Autodesk Inventor part; units mm, degrees
ref_plane "Work Plane1" through (5.1, 0, 0) normal (0, 0.866, -0.5) x (-1, 0, 0)
ref_plane "YZ Plane" through (0, 0, 0) normal (1, 0, 0) x (0, 1, 0)
ref_plane "XZ Plane" through (0, 0, 0) normal (0, 1, 0) x (-1, 0, 0)
sketch "Sketch1" plane through (0, 0, 0) normal (1, 0, 0) x (0, 1, 0)
  line L0 (-4.9075, -8.5) -> (-9.815, 0)
  line L1 (-9.815, 0) -> (-4.9075, 8.5)
  line L2 (-4.9075, 8.5) -> (4.9075, 8.5)
  line L3 (4.9075, 8.5) -> (9.815, 0)
  line L4 (9.815, 0) -> (4.9075, -8.5)
  line L5 (4.9075, -8.5) -> (-4.9075, -8.5)
  point P0 (0, 0)
  point P1 (0, 0)
  dimension "d0" = 19.6299
extrude "Body" add sketch "Sketch1" along normal blind 8
sketch "Sketch2" plane through (0, 0, 0) normal (0, 0, 1) x (1, 0, 0)
  line L0 (8, 0) -> (16.5, 0)
  arc A0 (16.5, 0) -> (8, 8.5) centre (8, 0) ccw
  line L1 (8, 8.5) -> (8, 8.5)
  line L2 (8, -4.9075) -> (8, 4.9075)
  line L3 (8, 0) -> (8, 8.5)
  line L4 (5.9479, 0) -> (20.3125, 0)
  dimension "d8" = 8.5
  dimension "d9" = 8.5
revolve "Cap" add sketch "Sketch2" angle 360 about axis through (8, 0, 0) along (1, 0, 0)
sketch "Sketch3" plane through (0, 0, 0) normal (-1, 0, 0) x (0, 0, 1)
  line L0 (0, -13.7409) -> (0, 13.7409)
  line L1 (-11.9, 0) -> (11.9, 0)
  point P0 (0, 0)
hole "Thread" at (0, 0, 0) direction (1, 0, 0) diameter 8.376 depth 10.2 tip angle 120
sketch "Sketch4" plane through (0, 0, 0) normal (0, 0, 1) x (1, 0, 0)
  line L0 (0, 4.9075) -> (0, 9.815)
  line L1 (0, 9.815) -> (8, 9.815)
  line L2 (8, 4.9075) -> (8, 9.815)
  line L3 (-1.6, 0) -> (9.6, 0)
  line L4 (0.7592, 9.815) -> (0, 8.5)
  line L5 (7.2408, 9.815) -> (8, 8.5)
  dimension "d3" = 17
  dimension "d4" = 30
  dimension "d5" = 17
  dimension "d6" = 30
revolve "Chamfer1" cut sketch "Sketch4" angle 360 about axis through (-10, 0, 0) along (1, 0, 0)
chamfer "Chamfer2" distance 0.8119 angle 30 1 edges at (0, 0, -4.188) measured on face at (0, -7.0214, 0.1683)
ref_plane "Work Plane1" through (5.1, 0, 0) normal (0, 0.866, -0.5) x (-1, 0, 0)
equation "\"d0\" = 1.1547 * SW"
equation "\"d1\" = SIH"
equation "\"d8\" = KR"
equation "\"d9\" = KOH1 - SIH"
equation "\"d11\" = GEL"
equation "\"d12\" = 1.02 * GEL"
equation "\"d3\" = SW0"
equation "\"d4\" = ANG1"
equation "\"d5\" = SW01"
equation "\"d6\" = ANG2"
equation "\"d14\" = -0.5 * GD1 + 0.5 * NND"
equation "\"d36\" = -0.5 * GD1 + 0.5 * NND"
equation "\"ANG1\" = 30deg"
equation "\"ANG2\" = ANG1"
equation "\"SIH\" = 8"
equation "\"KOH1\" = 16.5"
equation "\"GEL\" = 10"
equation "\"SW\" = 17"
equation "\"KR\" = 8.5"
equation "\"SW0\" = SW"
equation "\"SW01\" = SW"
equation "\"GUL\" = 0.541266 * PTC"
equation "\"TOA\" = 30deg"
equation "\"PTC\" = 1.5"
equation "\"E0\" = 1.155 * SW"
equation "\"GAL\" = 0.541266 * PTC"
properties part number "NF E 27-453 - M10" material "Steel, Mild"
Input: part model. Units: mm. Frame: model coordinates. Give positions to 0.01 mm unless a question says otherwise; leave off trailing zeros. Loops run counter-clockwise (first coordinate to the right, second up) from the corner with the lowest first, then second, coordinate; pieces in that order, holes last.
1) Contact query for flat-ended pins moving along their axis: pin 1 (6 mm diameter, centred on x = 11.5, y = -6.5, fed in from +Z); pin 2 (6 mm diameter, centred on x = 11, y = 0, fed in from +Z); pin 3 (1 mm diameter, centred on y = 5.5, z = 5, fed in from +X); pin 4 (6 mm diameter, centred on x = 10.5, z = -2.5, fed in from -Y). Output: stop coordinate, or through.
A:
pin 1: stops at z = 7.28
pin 2: stops at z = 8.5
pin 3: stops at x = 12.92
pin 4: stops at y = -8.95
2) Section query A-A on x = 7.5. Return the cut outline in (y, z).
A:
outline: (-9.33, -0.84) - (-5.39, -7.66) arc R9.37 ccw to (-3.93, -8.5) - (3.93, -8.5) arc R9.37 ccw to (5.39, -7.66) - (9.33, -0.84) arc R9.37 ccw to (9.33, 0.84) - (5.39, 7.66) arc R9.37 ccw to (3.93, 8.5) - (-3.93, 8.5) arc R9.37 ccw to (-5.39, 7.66) - (-9.33, 0.84) arc R9.37 ccw to start; hole circle Ø8.38 at (0, 0)
3) Mould query, pull axis Z, two halves, no side actions, for faces 1 (the cylindrical face through (5.402, -2.83, -3.087)), 2 (the conical face through (12.2, 0.22, 0.69)), 3 (the conical face through (7.87, 8.72, 0.19)), 4 (the flat face through (3.944, -7.327, -4.309)). Classes: released by +Z, released by -Z, zero draft, split by the parting line, or undercut.
A:
face 1: undercut
face 2: undercut
face 3: split by the parting line
face 4: released by -Z
4) Line query: L1, parallel to Z at x = 2.5, y = 0; L2, parallel to Z at x = 3.5, y = -3; L3, parallel to X at y = 0.5, z = 7.75. Output: solid intervals per line, ascending.
A:
L1: z = -8.5 to -4.19, 4.19 to 8.5
L2: z = -8.5 to -2.92, 2.92 to 8.5
L3: x = 0 to 11.46
5) Section query B-B on x = 14.5. Return the cut outline in (y, z).
A:
outline: circle Ø10.95 at (0, 0)
